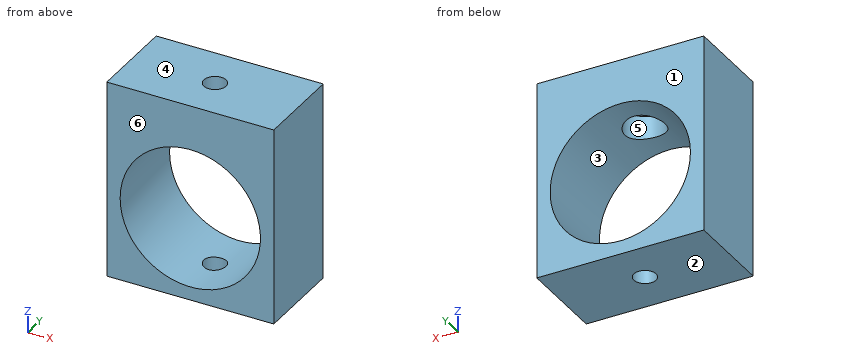
Autodesk Inventor part; units mm, degrees
ref_plane "YZ Plane" through (0, 0, 0) normal (1, 0, 0) x (0, 1, 0)
ref_plane "XZ Plane" through (0, 0, 0) normal (0, 1, 0) x (-1, 0, 0)
ref_plane "XY Plane" through (0, 0, 0) normal (0, 0, 1) x (1, 0, 0)
sketch "Sketch1" plane through (0, 0, 0) normal (0, 1, 0) x (-1, 0, 0)
  line L0 (0, 0) -> (-37.5, 0)
  line L1 (-37.5, 0) -> (-37.5, 37.5)
  line L2 (-37.5, 37.5) -> (0, 37.5)
  line L3 (0, 37.5) -> (0, 0)
  circle A0 centre (-18.75, 18.75) radius 15.75
  point P0 (-18.75, 0)
  dimension "d0" = 37.5
  dimension "d1" = 37.5
  dimension "d2" = 18.75
  dimension "d3" = 18.75
  dimension "d4" = 31.5
extrude "Extrusion1" add sketch "Sketch1" against normal blind 20
sketch "Sketch3" plane through (0, 0, 37.5) normal (0, 0, 1) x (1, 0, 0)
  circle A0 centre (18.75, -10) radius 4.5
  line L0 (37.5, 0) -> (37.5, -20)
  point P0 (0, 0)
  point P1 (37.5, -10)
  dimension "d8" = 9
  dimension "d19" = 18.75
extrude "Extrusion2" cut sketch "Sketch3" against normal blind 5
sketch "Sketch4" plane through (37.5, 0, 0) normal (0, 0, -1) x (-1, 0, 0)
  circle A0 centre (18.75, -10) radius 4.5
  circle A1 centre (18.75, -10) radius 2.5
  point P0 (37.5, 0)
  dimension "d11" = 5
extrude "Extrusion3" cut sketch "Sketch4" against normal blind 5 contours A1
sketch "Sketch5" plane through (0, 0, 37.5) normal (0, 0, 1) x (1, 0, 0)
  line L0 (37.5, 0) -> (0, 0)
  line L1 (0, -20) -> (37.5, -20)
  line L2 (0, 0) -> (37.5, 0)
  line L3 (37.5, 0) -> (37.5, -20)
  line L4 (37.5, -20) -> (0, -20)
  line L5 (0, -20) -> (0, 0)
  line L6 (0, 0) -> (0, -20)
  line L7 (0, 0) -> (37.5, 0)
  line L8 (37.5, 0) -> (37.5, -20)
  line L9 (37.5, -20) -> (0, -20)
  line L10 (0, -20) -> (0, 0)
  circle A0 centre (18.75, -10) radius 4.5
  point P0 (37.5, -10)
  dimension "d18" = 18.75
extrude "Extrusion4" add sketch "Sketch5" along normal blind 2
sketch "Sketch6" plane through (0, 0, 39.5) normal (0, 0, 1) x (1, 0, 0)
  line L0 (0, 0) -> (0, -20)
  line L1 (0, -20) -> (37.5, -20)
  line L2 (0, 0) -> (37.5, 0)
  line L3 (37.5, 0) -> (37.5, -20)
  line L4 (37.5, -20) -> (0, -20)
  line L5 (0, -20) -> (0, 0)
  circle A0 centre (18.75, -10) radius 2.5
  dimension "d20" = 18.75
extrude "Extrusion5" add sketch "Sketch6" along normal blind 5
equation "\"d0\" = d1"
properties part number "welco mount v04"
Design review of the part built by this model. Coordinates are the model's own, in mm. Face numbers are marked on the shaded views. A direction names the side the tool comes from. Round coordinates to 2 decimals unless told otherwise and drop trailing zeros. Order: outer loops, then holes, each group sorted by start corner. A loop starts at its lowest first (then second) coordinate and runs counter-clockwise, first axis right, second up.
1) Machinability: for the marked faces 5 and 6, which of the approach directions +Z, -Z, +X, -X, +Y, -Y give a long, thin tool a straight path to every point of the face, cutting with its end or side? Answer none if there is none.
The answers:
face 5: none
face 6: +Z, -Z, +X, -X, -Y
2) Consider section C-C (y = -10). State the section outline as (x, z) points.
The answers:
outline: (0, 0) - (16.25, 0) - (16.25, 3.2) arc R15.75 cw to (14.25, 33.84) - (14.25, 39.5) - (16.25, 39.5) - (16.25, 44.5) - (0, 44.5) - close; (21.25, 0) - (37.5, 0) - (37.5, 44.5) - (21.25, 44.5) - (21.25, 39.5) - (23.25, 39.5) - (23.25, 33.84) arc R15.75 cw to (21.25, 3.2) - close
3) Clearance check with a flat-ended pin moving along its axis: pin 1 Ø4.5 at (x, y) = (18.75, -10) entering from -Z. State where the tip first meets the part, or that it passes through.
The answers:
pin 1: passes through
4) Consider section B-B (z = 18.75). State the section outline as (x, y) points, plus the area to 3 significant figures.
The answers:
outline: (0, -20) - (3, -20) - (3, 0) - (0, 0) - close; (34.5, -20) - (37.5, -20) - (37.5, 0) - (34.5, 0) - close
area: 120 mm2
5) Draft analysis for pull direction Z (two halves, no side actions). For the marked faces 1, 2, 3 and 4, state which applies: released by +Z, released by -Z, zero draft, split by the parting line, or undercut.
The answers:
face 1: zero draft
face 2: released by -Z
face 3: undercut
face 4: released by +Z
6) Consider section D-D (x = 5). State the section outline as (y, z) points, plus the area to 3 significant figures.
The answers:
outline: (-20, 0) - (0, 0) - (0, 11.07) - (-20, 11.07) - close; (-20, 26.43) - (0, 26.43) - (0, 44.5) - (-20, 44.5) - close
area: 583 mm2
7) Consider section A-A (x = 18.75). State the section outline as (y, z) points, plus the area to 3 significant figures.
The answers:
outline: (-20, 0) - (-12.5, 0) - (-12.5, 3) - (-20, 3) - close; (-20, 34.5) - (-14.5, 34.5) - (-14.5, 39.5) - (-12.5, 39.5) - (-12.5, 44.5) - (-20, 44.5) - close; (-7.5, 0) - (0, 0) - (0, 3) - (-7.5, 3) - close; (-7.5, 39.5) - (-5.5, 39.5) - (-5.5, 34.5) - (0, 34.5) - (0, 44.5) - (-7.5, 44.5) - close
area: 175 mm2
8) For L1, parallel to X at y = -10, z = 2.1; L2, parallel to Y at x = 22.5, z = 37; L3, parallel to Y at x = 18.75, z = 35.25, list the stretches that pass through material, from the lowest coordinate up.
The answers:
L1: x = 0 to 16.25, 21.25 to 37.5
L2: y = -20 to -12.49, -7.51 to 0
L3: y = -20 to -14.5, -5.5 to 0
